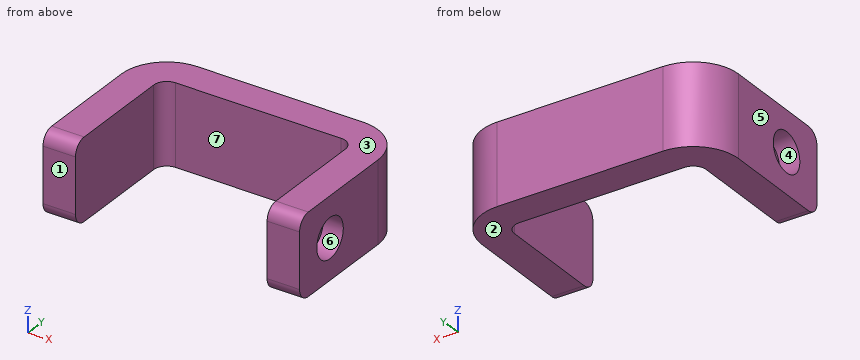
```python
from build123d import *

# Parameters (mm, degrees)
BOSS_EXTRUDE1_DEPTH = 6.25
SKETCH2_R           = 3.05
CUT_EXTRUDE1_DEPTH  = 3.1
FILLET1_R           = 2
FILLET2_R           = 7
FILLET3_R           = 2


with BuildPart() as part:
    # Sketch1 → Boss-Extrude1 (new body, symmetric)
    with BuildSketch(Plane.XY):
        Polygon((-14.75, 0), (-19.75, 0), (-19.75, 25), (19.75, 25), (19.75, 0), (14.75, 0), (14.75, 20), (-14.75, 20), align=None)
    extrude(amount=BOSS_EXTRUDE1_DEPTH, both=True)

    # Sketch2 → Cut-Extrude1 (cut)
    with BuildSketch(Plane.ZY.offset(19.75)):
        with Locations((0, 7)):
            Circle(SKETCH2_R)
    cut_extrude1 = extrude(amount=-CUT_EXTRUDE1_DEPTH, mode=Mode.SUBTRACT)

    # Mirror1: Cut-Extrude1 across plane
    add(cut_extrude1.mirror(Plane(origin=(0, 0, 0), x_dir=(0, 0, 1), z_dir=(1, 0, 0))), mode=Mode.SUBTRACT)

    # Fillet1
    fillet1_edges = [part.edges().sort_by_distance(p)[0] for p in [
        (14.75, 20, 0),
        (-14.75, 20, 0),
    ]]
    fillet(fillet1_edges, radius=FILLET1_R)

    # Fillet2
    fillet2_edges = [part.edges().sort_by_distance(p)[0] for p in [
        (-19.75, 25, 0),
        (19.75, 25, 0),
    ]]
    fillet(fillet2_edges, radius=FILLET2_R)

    # Fillet3
    fillet3_edges = [part.edges().sort_by_distance(p)[0] for p in [
        (17.25, 0, -6.25),
        (17.25, 0, 6.25),
        (-17.25, 0, 6.25),
        (-17.25, 0, -6.25),
    ]]
    fillet(fillet3_edges, radius=FILLET3_R)


solid = part.part
```
Can you work these out from the model? Positions are in its coordinate system, mm. Face numbers are marked on the shaded views. A direction names the side the tool comes from. Coordinates: 2 decimals unless noted, no trailing zeros. Loops run counter-clockwise (first coordinate to the right, second up) from the corner with the lowest first, then second, coordinate; pieces in that order, holes last.
1) Thinking about a two-plate mould opening in Z: for the marked faces 1, 2, 3 and 4, which applies, pulls with the +Z half, pulls with the -Z half, needs draft (parallel to the pull), parting line crosses it, or undercut?
2) Imagine slicing it at C-C on y = 7. List the corners of the cut face in (x, z) for me, plus the area to 3 significant figures.
3) Imagine slicing it at D-D on x = 1.5. List the corners of the cut face in (y, z) for me, plus the area to 3 significant figures.
4) I need wall thicknesses on probe 1 along X at (y, z) = (17.5, 0.5); probe 2 along X at (y, z) = (5, 1.75); probe 3 along Y at (x, z) = (0, 5.5). Which ranges of each line are inside material? Lowest first, please.
5) For pin 1 (3 mm diameter, centred on x = 13, z = -3, fed in from -Y); pin 2 (3.5 mm diameter, centred on y = 7, z = 0, fed in from +X); pin 3 (4 mm diameter, centred on y = 7.5, z = -2, fed in from -X); pin 4 (1.8 mm diameter, centred on y = 7, z = -1.5, fed in from -X), each with a flat end and sliding along its axis, tell me the tip position at first contact or that it passes through.
6) Which directions (+Z, -Z, +X, -X, +Y, -Y) give clear straight access to the entire face, cutting with the end or side of a thin tool? Please do the marked faces 5, 6 and 7.
7) Imagine slicing it at B-B on z = -3.75. List the corners of the cut face in (x, y) for me, plus the area to 3 significant figures.
8) Imagine slicing it at A-A on y = 12.5. List the corners of the cut face in (x, z) for me.
Completed:
1. face 1: needs draft
1. face 2: pulls with the -Z half
1. face 3: pulls with the +Z half
1. face 4: undercut
2. outline: (-19.75, -6.25) - (-14.75, -6.25) - (-14.75, 6.25) - (-19.75, 6.25) - (-19.75, 3.05) - (-16.65, 3.05) - (-16.65, -3.05) - (-19.75, -3.05) - close; (14.75, -6.25) - (19.75, -6.25) - (19.75, -3.05) - (16.65, -3.05) - (16.65, 3.05) - (19.75, 3.05) - (19.75, 6.25) - (14.75, 6.25) - close
2. area: 87.2 mm2
3. outline: (20, -6.25) - (25, -6.25) - (25, 6.25) - (20, 6.25) - close
3. area: 62.5 mm2
4. probe 1: x = -19.75 to -14.75, 14.75 to 19.75
4. probe 2: x = -16.65 to -14.75, 14.75 to 16.65
4. probe 3: y = 20 to 25
5. pin 1: stops at y = 18.97
5. pin 2: stops at x = 16.65
5. pin 3: stops at x = -19.75
5. pin 4: stops at x = -16.65
6. face 5: +Z, -Z, -X, +Y, -Y
6. face 6: +X
6. face 7: +Z, -Z, -Y
7. outline: (-19.75, 0) - (-14.75, 0) - (-14.75, 18) arc R2 cw to (-12.75, 20) - (12.75, 20) arc R2 cw to (14.75, 18) - (14.75, 0) - (19.75, 0) - (19.75, 18) arc R7 ccw to (12.75, 25) - (-12.75, 25) arc R7 ccw to (-19.75, 18) - close
7. area: 378 mm2
8. outline: (-19.75, -6.25) - (-14.75, -6.25) - (-14.75, 6.25) - (-19.75, 6.25) - close; (14.75, -6.25) - (19.75, -6.25) - (19.75, 6.25) - (14.75, 6.25) - close
